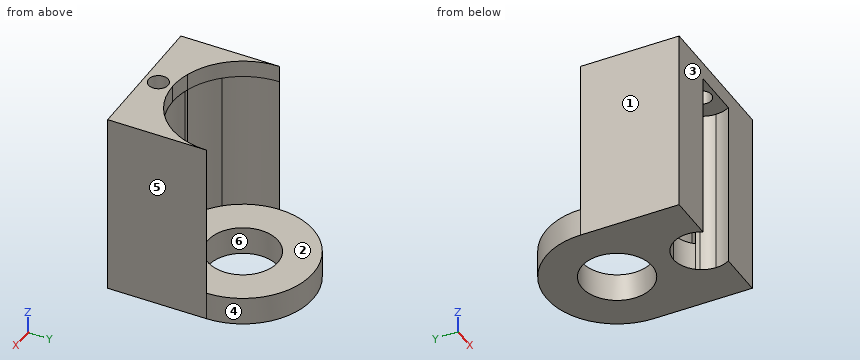
```python
from build123d import *

# Parameters (mm, degrees)
F1_DEPTH = 5
F2_DEPTH = 30
F3_R     = 1.75
F4_DEPTH = 3


with BuildPart() as f1:
    # F0 (on Top) → F1 (new body)
    with BuildSketch(Plane.XY):
        with BuildLine():
            Line((6.25, 0), (10, 0))
            ThreePointArc((10, 0), (0, 10), (-10, 0))
            Line((-10, 0), (-6.25, 0))
            ThreePointArc((-6.25, 0), (0, 6.25), (6.25, 0))
        make_face()
        with BuildLine():
            Line((12.5, 0), (10, 0))
            ThreePointArc((10, 0), (8.7372269275, -4.8642435813), (5.2678268764, -8.5))
            Line((5.2678268764, -8.5), (9.1651513899, -8.5))
            ThreePointArc((9.1651513899, -8.5), (11.6364597789, -4.5653919671), (12.5, 0))
        make_face()
        with BuildLine():
            ThreePointArc((5.2678268764, -8.5), (8.7372269275, -4.8642435813), (10, 0))
            Line((10, 0), (6.25, 0))
            ThreePointArc((6.25, 0), (0, -6.25), (-6.25, 0))
            Line((-6.25, 0), (-10, 0))
            ThreePointArc((-10, 0), (-8.7372269275, -4.8642435813), (-5.2678268764, -8.5))
            Line((-5.2678268764, -8.5), (5.2678268764, -8.5))
        make_face()
        with BuildLine():
            ThreePointArc((-10, 0), (0, 10), (10, 0))
            Line((10, 0), (12.5, 0))
            ThreePointArc((12.5, 0), (0, 12.5), (-12.5, 0))
            Line((-12.5, 0), (-10, 0))
        make_face()
        with BuildLine():
            ThreePointArc((-5.2678268764, -8.5), (-8.7372269275, -4.8642435813), (-10, 0))
            Line((-10, 0), (-12.5, 0))
            ThreePointArc((-12.5, 0), (-11.6364597789, -4.5653919671), (-9.1651513899, -8.5))
            Line((-9.1651513899, -8.5), (-5.2678268764, -8.5))
        make_face()
        with BuildLine():
            Line((9.1651513899, -8.5), (5.2678268764, -8.5))
            ThreePointArc((5.2678268764, -8.5), (2.7386127875, -9.6176920308), (0, -10))
            ThreePointArc((0, -10), (2.1650635095, -10.4930609057), (3.903123749, -11.875))
            ThreePointArc((3.903123749, -11.875), (6.7485265078, -10.5217579317), (9.1651513899, -8.5))
        make_face()
        with BuildLine():
            ThreePointArc((0, -10), (2.7386127875, -9.6176920308), (5.2678268764, -8.5))
            Line((5.2678268764, -8.5), (-5.2678268764, -8.5))
            ThreePointArc((-5.2678268764, -8.5), (-2.7386127875, -9.6176920308), (0, -10))
        make_face()
        with BuildLine():
            ThreePointArc((0, -10), (-2.7386127875, -9.6176920308), (-5.2678268764, -8.5))
            Line((-5.2678268764, -8.5), (-9.1651513899, -8.5))
            ThreePointArc((-9.1651513899, -8.5), (-6.7485265078, -10.5217579317), (-3.903123749, -11.875))
            ThreePointArc((-3.903123749, -11.875), (-2.1650635095, -10.4930609057), (0, -10))
        make_face()
    extrude(amount=F1_DEPTH)

    # F0 (on Top) → F2 (join)
    with BuildSketch(Plane.XY):
        with BuildLine():
            ThreePointArc((-9.1651513899, -8.5), (-11.6364597789, -4.5653919671), (-12.5, 0))
            Line((-12.5, 0), (-12.5, -8.5))
            Line((-12.5, -8.5), (-9.1651513899, -8.5))
        make_face()
        with BuildLine():
            Line((12.5, -8.5), (12.5, 0))
            ThreePointArc((12.5, 0), (11.6364597789, -4.5653919671), (9.1651513899, -8.5))
            Line((9.1651513899, -8.5), (12.5, -8.5))
        make_face()
        with BuildLine():
            Line((12.5, -8.5), (9.1651513899, -8.5))
            ThreePointArc((9.1651513899, -8.5), (6.7485265078, -10.5217579317), (3.903123749, -11.875))
            ThreePointArc((3.903123749, -11.875), (4.1284695472, -12.1794080057), (4.3301270189, -12.5))
            Line((4.3301270189, -12.5), (12.5, -12.5))
            Line((12.5, -12.5), (12.5, -8.5))
        make_face()
        with BuildLine():
            ThreePointArc((-3.903123749, -11.875), (-6.7485265078, -10.5217579317), (-9.1651513899, -8.5))
            Line((-9.1651513899, -8.5), (-12.5, -8.5))
            Line((-12.5, -8.5), (-12.5, -12.5))
            Line((-12.5, -12.5), (-4.3301270189, -12.5))
            ThreePointArc((-4.3301270189, -12.5), (-4.1284695472, -12.1794080057), (-3.903123749, -11.875))
        make_face()
        with BuildLine():
            Line((-4.3301270189, -12.5), (-12.5, -12.5))
            Line((-12.5, -12.5), (-12.5, -17.5))
            Line((-12.5, -17.5), (-4.3301270189, -17.5))
            ThreePointArc((-4.3301270189, -17.5), (-5, -15), (-4.3301270189, -12.5))
        make_face()
        with BuildLine():
            Line((12.5, -17.5), (12.5, -12.5))
            Line((12.5, -12.5), (4.3301270189, -12.5))
            ThreePointArc((4.3301270189, -12.5), (4.8296291314, -13.7059047745), (5, -15))
            ThreePointArc((5, -15), (4.8296291314, -16.2940952255), (4.3301270189, -17.5))
            Line((4.3301270189, -17.5), (12.5, -17.5))
        make_face()
    extrude(amount=F2_DEPTH)

    # F3 (on face) → F4 (join)
    with BuildSketch(Plane.XY.offset(30)):
        with BuildLine():
            Line((0, -12.5), (-4.3301270189, -12.5))
            ThreePointArc((-4.3301270189, -12.5), (-5, -15), (-4.3301270189, -17.5))
            Line((-4.3301270189, -17.5), (12.5, -17.5))
            Line((12.5, -17.5), (12.5, -12.5))
            Line((12.5, -12.5), (0, -12.5))
        make_face()
        with Locations((0, -15)):
            Circle(F3_R, mode=Mode.SUBTRACT)
        with BuildLine():
            ThreePointArc((-3.903123749, -11.875), (-10.1251925133, -7.3301075414), (-12.5, 0))
            Line((-12.5, 0), (-12.5, -12.5))
            Line((-12.5, -12.5), (-4.3301270189, -12.5))
            ThreePointArc((-4.3301270189, -12.5), (-4.1284695472, -12.1794080057), (-3.903123749, -11.875))
        make_face()
        with BuildLine():
            Line((-4.3301270189, -12.5), (-12.5, -12.5))
            Line((-12.5, -12.5), (-12.5, -17.5))
            Line((-12.5, -17.5), (-4.3301270189, -17.5))
            ThreePointArc((-4.3301270189, -17.5), (-5, -15), (-4.3301270189, -12.5))
        make_face()
        with BuildLine():
            Line((12.5, -12.5), (12.5, 0))
            ThreePointArc((12.5, 0), (8.8388347648, -8.8388347648), (0, -12.5))
            Line((0, -12.5), (12.5, -12.5))
        make_face()
        with BuildLine():
            ThreePointArc((0, -12.5), (-1.9764235376, -12.3427610363), (-3.903123749, -11.875))
            ThreePointArc((-3.903123749, -11.875), (-4.1284695472, -12.1794080057), (-4.3301270189, -12.5))
            Line((-4.3301270189, -12.5), (0, -12.5))
        make_face()
    extrude(amount=F4_DEPTH)


solid = f1.part
```
Geometry: final body of the model. Coordinates: model frame, mm. Face numbers are marked on the shaded views. A direction names the side the tool comes from. Coordinates: 2 decimals unless noted, no trailing zeros. Loops run counter-clockwise (first coordinate to the right, second up) from the corner with the lowest first, then second, coordinate; pieces in that order, holes last. Notation, with made-up numbers: (59, 44.5) -> (71, 44.5) arc R5 cw to (71, 53.5) -> close; hole circle Ø9 at (46.5, 39.25). An arc over 180 degrees is marked (long way). Use a Markdown table: item, result. Add a question column.
(1) Section query D-D, the plane x = -5.5. Return loops of the section in (y, z).
(2) Access query for the marked faces 1 and 2. Directions: +Z, -Z, +X, -X, +Y, -Y. A direction counts if a zero-diameter tool reaches every point of the face in a straight line with its end or side. Return the directions, or none.
(3) Line query: line 1 along Y through (x, z) = (0, 32.4); line 2 along Y through (x, z) = (0, 1.1); line 3 along X through (y, z) = (-8.5, 29.5). Output: solid intervals per line, ascending.
(4) Section query B-B, the plane z = 19.5. Return loops of the section in (x, y) (3 decimals).
(5) Section query A-A, the plane z = 4. Return loops of the section in (x, y) (3 decimals), plus the area to 3 significant figures.
(6) Section query C-C, the plane y = -5.5. Return loops of the section in (x, z), plus the area to 3 significant figures.
(7) Mould query, pull axis Y, two halves, no side actions, for the marked faces 3, 4, 5 and 6. Classes: pulls with the +Y half, pulls with the -Y half, needs draft (parallel to the pull), parting line crosses it, or undercut.
(8) Pin query (flat end, axial travel): pin 1 Ø6 at (x, y) = (6, 3.5) entering from +Z; pin 2 Ø7.5 at (x, y) = (0, 0) entering from -Z; pin 3 Ø6 at (x, y) = (1, -15) entering from -Z; pin 4 Ø10 at (y, z) = (5.5, 9.5) entering from -X. Return the tip coordinate at first contact, or that it passes through.
Answer:
| question | item | result |
|---|---|---|
| 1 | outline | (-17.5, 0) -> (-2.97, 0) -> (-2.97, 5) -> (-11.22, 5) -> (-11.22, 33) -> (-17.5, 33) -> close; (2.97, 0) -> (11.22, 0) -> (11.22, 5) -> (2.97, 5) -> close |
| 2 | face 1 | +Z, -Z, -X, +Y, -Y |
| 2 | face 2 | +Z, +Y |
| 3 | line 1 | y = -17.5 to -16.75, -13.25 to -12.5 |
| 3 | line 2 | y = -10 to -6.25, 6.25 to 12.5 |
| 3 | line 3 | x = -12.5 to -9.17, 9.17 to 12.5 |
| 4 | outline | (-12.5, -17.5) -> (-4.33, -17.5) arc R5 cw to (-3.903, -11.875) arc R12.5 cw to (-12.5, 0) -> close; (3.903, -11.875) arc R5 cw to (4.33, -17.5) -> (12.5, -17.5) -> (12.5, 0) arc R12.5 cw to start |
| 5 | outline | (-12.5, -17.5) -> (-4.33, -17.5) arc R5 cw (long way) to (4.33, -17.5) -> (12.5, -17.5) -> (12.5, 0) arc R12.5 ccw to (-12.5, 0) -> close; hole circle Ø12.5 at (0, 0) |
| 5 | area | 497 mm^2 |
| 6 | outline | (-12.5, 0) -> (-2.97, 0) -> (-2.97, 5) -> (-11.22, 5) -> (-11.22, 33) -> (-12.5, 33) -> close; (2.97, 0) -> (12.5, 0) -> (12.5, 33) -> (11.22, 33) -> (11.22, 5) -> (2.97, 5) -> close |
| 6 | area | 167 mm^2 |
| 7 | face 3 | pulls with the -Y half |
| 7 | face 4 | pulls with the +Y half |
| 7 | face 5 | needs draft |
| 7 | face 6 | undercut |
| 8 | pin 1 | stops at z = 5 |
| 8 | pin 2 | passes through |
| 8 | pin 3 | stops at z = 30 |
| 8 | pin 4 | stops at x = -12.05 |
